Verification items for the finished model (mm, model axes). Coordinates: 2 decimals unless noted, no trailing zeros. Return JSON: item names as keys, results as strings. Group by question number.
1. Material ranges on line 1 along Z through (x, y) = (298.5, 13.8); line 2 along Z through (x, y) = (283.5, 12.8); line 3 along Z through (x, y) = (-256, -12.75), recorded low to high.
2. Gauge pin test, flat ends, axial feed: pin 1 (3 mm diameter, centred on x = -283.5, y = 0, fed in from -Z); pin 2 (5 mm diameter, centred on x = 198.5, z = 6, fed in from +Y); pin 3 (1 mm diameter, centred on y = 9, z = 1, fed in from -X); pin 4 (1.5 mm diameter, centred on x = 126, z = 6, fed in from -Y). Record the tip position at first contact, or that the pin passes through.
3. Section check A-A, the plane x = 110.5. Give the number of separate pieces and of enclosed holes in the cut face, plus the area to 3 significant figures.
```python
from build123d import *

# Parameters (mm, degrees)
SKETCH_1_W             = 23.5
SKETCH_1_H             = 12
EXTRUDE_1_DEPTH        = 318.5
HOLE_WIZARD_M6_1_D     = 5
HOLE_WIZARD_M6_1_DEPTH = 15
HOLE_WIZARD_M6_1_TIP   = 1.502151548
HOLE_WIZARD_M6_2_D     = 5
HOLE_WIZARD_M6_2_DEPTH = 15
HOLE_WIZARD_M6_2_TIP   = 1.502151548
HOLE_WIZARD_M4_1_D     = 3.3
HOLE_WIZARD_M4_1_DEPTH = 10.1
HOLE_WIZARD_M4_1_TIP   = 0.991420021


with BuildPart() as part:
    # 草图1 → 凸台-拉伸1 (new, symmetric)
    with BuildSketch(Plane(origin=(0, 0, 0), x_dir=(0, 0, -1), z_dir=(1, 0, 0))):
        with BuildLine():
            Line((-14, 15), (-11.5, 15))
            Line((-11.5, 15), (-11.5, 13.5))
            Line((-11.5, 13.5), (-11.4, 13.5))
            ThreePointArc((-11.4, 13.5), (-11.117157288, 13.382842712), (-11, 13.1))
            Line((-11, 13.1), (-11, 12))
            Line((-11, 12), (-9.5, 12))
            Line((-9.5, 12), (-9.5, 15))
            Line((-9.5, 15), (-8, 15))
            Line((-8, 15), (-8, 12.5))
            Line((-8, 12.5), (-5, 12.5))
            Line((-5, 12.5), (-5, 15))
            Line((-5, 15), (5, 15))
            Line((5, 15), (5, 12.5))
            Line((5, 12.5), (8, 12.5))
            Line((8, 12.5), (8, 15))
            Line((8, 15), (9.5, 15))
            Line((9.5, 15), (9.5, 12))
            Line((9.5, 12), (11, 12))
            Line((11, 12), (11, 13.1))
            ThreePointArc((11, 13.1), (11.117157288, 13.382842712), (11.4, 13.5))
            Line((11.4, 13.5), (11.5, 13.5))
            Line((11.5, 13.5), (11.5, 15))
            Line((11.5, 15), (14, 15))
            ThreePointArc((14, 15), (14.707106781, 14.707106781), (15, 14))
            Line((15, 14), (15, 8))
            Line((15, 8), (12.5, 8))
            Line((12.5, 8), (12.5, 5))
            Line((12.5, 5), (15, 5))
            Line((15, 5), (15, -5))
            Line((15, -5), (12.5, -5))
            Line((12.5, -5), (12.5, -8))
            Line((12.5, -8), (15, -8))
            Line((15, -8), (15, -14))
            ThreePointArc((15, -14), (14.707106781, -14.707106781), (14, -15))
            Line((14, -15), (11.5, -15))
            Line((11.5, -15), (11.5, -13.5))
            Line((11.5, -13.5), (11.4, -13.5))
            ThreePointArc((11.4, -13.5), (11.117157288, -13.382842712), (11, -13.1))
            Line((11, -13.1), (11, -12))
            Line((11, -12), (9.5, -12))
            Line((9.5, -12), (9.5, -15))
            Line((9.5, -15), (8, -15))
            Line((8, -15), (8, -12.5))
            Line((8, -12.5), (5, -12.5))
            Line((5, -12.5), (5, -15))
            Line((5, -15), (-5, -15))
            Line((-5, -15), (-5, -12.5))
            Line((-5, -12.5), (-8, -12.5))
            Line((-8, -12.5), (-8, -15))
            Line((-8, -15), (-9.5, -15))
            Line((-9.5, -15), (-9.5, -12))
            Line((-9.5, -12), (-11, -12))
            Line((-11, -12), (-11, -13.1))
            ThreePointArc((-11, -13.1), (-11.117157288, -13.382842712), (-11.4, -13.5))
            Line((-11.4, -13.5), (-11.5, -13.5))
            Line((-11.5, -13.5), (-11.5, -15))
            Line((-11.5, -15), (-14, -15))
            ThreePointArc((-14, -15), (-14.707106781, -14.707106781), (-15, -14))
            Line((-15, -14), (-15, 14))
            ThreePointArc((-15, 14), (-14.707106781, 14.707106781), (-14, 15))
        make_face()
        with BuildLine():
            Line((12, -10.5), (12, -8.5))
            ThreePointArc((12, -8.5), (11.853553391, -8.146446609), (11.5, -8))
            Line((11.5, -8), (-11.5, -8))
            ThreePointArc((-11.5, -8), (-11.853553391, -8.146446609), (-12, -8.5))
            Line((-12, -8.5), (-12, -10.5))
            ThreePointArc((-12, -10.5), (-11.853553391, -10.853553391), (-11.5, -11))
            Line((-11.5, -11), (11.5, -11))
            ThreePointArc((11.5, -11), (11.853553391, -10.853553391), (12, -10.5))
        make_face(mode=Mode.SUBTRACT)
        with BuildLine():
            Line((-11.5, 11), (11.5, 11))
            ThreePointArc((11.5, 11), (11.853553391, 10.853553391), (12, 10.5))
            Line((12, 10.5), (12, 8.5))
            ThreePointArc((12, 8.5), (11.853553391, 8.146446609), (11.5, 8))
            Line((11.5, 8), (-11.5, 8))
            ThreePointArc((-11.5, 8), (-11.853553391, 8.146446609), (-12, 8.5))
            Line((-12, 8.5), (-12, 10.5))
            ThreePointArc((-12, 10.5), (-11.853553391, 10.853553391), (-11.5, 11))
        make_face(mode=Mode.SUBTRACT)
        Rectangle(SKETCH_1_W, SKETCH_1_H, mode=Mode.SUBTRACT)
    extrude(amount=EXTRUDE_1_DEPTH, both=True)

    # M6 螺纹孔1
    with Locations(Plane(origin=(0, 15, 0), x_dir=(-1, 0, 0), z_dir=(0, 1, 0))):
        with Locations((298.5, 0), (283.5, 0), (-283.5, 0), (-298.5, 0)):
            Hole(HOLE_WIZARD_M6_1_D / 2, depth=HOLE_WIZARD_M6_1_DEPTH)
            with Locations((0, 0, -(HOLE_WIZARD_M6_1_DEPTH + HOLE_WIZARD_M6_1_TIP / 2))):  # 118° drill point
                Cone(0, HOLE_WIZARD_M6_1_D / 2, HOLE_WIZARD_M6_1_TIP, mode=Mode.SUBTRACT)

    # M6 螺纹孔2
    with Locations(Plane(origin=(0, 0, -15), x_dir=(-1, 0, 0), z_dir=(0, 0, -1))):
        with Locations((298.5, 0), (283.5, 0)):
            Hole(HOLE_WIZARD_M6_2_D / 2, depth=HOLE_WIZARD_M6_2_DEPTH)
            with Locations((0, 0, -(HOLE_WIZARD_M6_2_DEPTH + HOLE_WIZARD_M6_2_TIP / 2))):  # 118° drill point
                Cone(0, HOLE_WIZARD_M6_2_D / 2, HOLE_WIZARD_M6_2_TIP, mode=Mode.SUBTRACT)

    # M4 螺纹孔1
    with Locations(Plane(origin=(0, 0, -15), x_dir=(-1, 0, 0), z_dir=(0, 0, -1))):
        with Locations((-303.5, 0), (-118.5, 0), (1.5, 0), (98.5, 0), (248.5, 0)):
            Hole(HOLE_WIZARD_M4_1_D / 2, depth=HOLE_WIZARD_M4_1_DEPTH)
            with Locations((0, 0, -(HOLE_WIZARD_M4_1_DEPTH + HOLE_WIZARD_M4_1_TIP / 2))):  # 118° drill point
                Cone(0, HOLE_WIZARD_M4_1_D / 2, HOLE_WIZARD_M4_1_TIP, mode=Mode.SUBTRACT)


solid = part.part
```
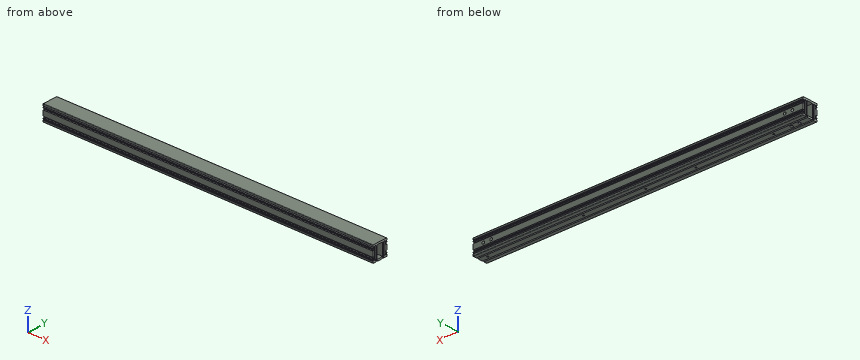
Answers follow:
{
 "1": {"line 1": "-15 to -11.5, -9.5 to -8, -5 to -2.5, 2.5 to 5, 8 to 9.5, 11.5 to 15", "line 2": "-15 to -11, -9.5 to -8, -5 to -2.5, 2.5 to 5, 8 to 9.5, 11 to 15", "line 3": "-15 to -11, -9.5 to -8, -5 to 5, 8 to 9.5, 11 to 15"},
 "2": {"pin 1": "z = 11.75", "pin 2": "y = 15", "pin 3": "through", "pin 4": "y = -12.5"},
 "3": {"separate pieces": "1", "enclosed holes": "3", "area": "407 mm^2"}
}
